from build123d import *

# Parameters (mm, degrees)
SKETCH_1_R          = 5
EXTRUDE_1_DEPTH     = 8.7
SKETCH_2_R          = 7
EXTRUDE_2_DEPTH     = 1.5
EXTRUDE_START       = -1.5
SKETCH_3_R          = 7
EXTRUDE_3_DEPTH     = 1.5
SKETCH_4_R          = 3
CUT_EXTRUDE_1_DEPTH = 10


with BuildPart() as part:
    # 草图1 → 凸台-拉伸1 (new body)
    with BuildSketch(Plane(origin=(0, 0, 0), x_dir=(0, 0, -1), z_dir=(1, 0, 0))):
        Circle(SKETCH_1_R)
    extrude(amount=EXTRUDE_1_DEPTH)

    # 草图2 → 凸台-拉伸2 (add)
    with BuildSketch(Plane(origin=(8.7, 0, 0), x_dir=(0, 0, -1), z_dir=(1, 0, 0))):
        Circle(SKETCH_2_R)
    extrude(amount=-EXTRUDE_2_DEPTH)

    # 草图3 → 凸台-拉伸3 (add)
    with BuildSketch(Plane.ZY.offset(EXTRUDE_START)):
        with Locations(Location((0, 0, 0), (0, 0, 180))):
            Circle(SKETCH_3_R)
    extrude(amount=EXTRUDE_3_DEPTH)

    # 草图4 → 切除-拉伸1 (cut)
    with BuildSketch(Plane(origin=(8.7, 0, 0), x_dir=(0, 0, -1), z_dir=(1, 0, 0))):
        Circle(SKETCH_4_R)
    extrude(amount=-CUT_EXTRUDE_1_DEPTH, mode=Mode.SUBTRACT)


solid = part.part
The listing builds one solid part. Answer for the finished solid, in the listing's coordinates (mm). A direction names the side the tool comes from. Give positions to 0.01 mm unless a question says otherwise; leave off trailing zeros. Write each loop counter-clockwise with the first axis right and the second up, starting at its lowest first coordinate (ties: lowest second). Pieces come first, ordered by that corner, then holes.
1) Section D-D (z = 3.75) is taken. Write down the section's boundary in (x, y).
2) Given P1, Ø5, axis at x = 6.5, z = 5, coming from the +Y side; P2, Ø3, axis at x = 6, y = 1.5, coming from the +Z side; P3, Ø1.5, axis at x = 2, z = 5.5, coming from the +Y side, each flat-ended and moving along its own axis, determine where each tip first touches the part or whether it passes through.
3) A tool of negligible diameter and unlimited length cuts with its end or side. For faces 4 (the face through (7.2, 5, 2)), 5 (the face through (0.76, 2.681, -6.466)), from which of +Z, -Z, +X, -X, +Y, -Y can it reach the whole face along a straight path? Write none if from no direction.
4) Section A-A (z = 0) is taken. Write down the section's boundary in (x, y), and give its area (3 significant figures).
5) Section C-C (x = 0.75) is taken. Write down the section's boundary in (y, z), and give its area (3 significant figures).
6) For a pull along Z with two mould halves and no side action, classify faces 1 (the face through (4.31, -4.88, 1.08)), 2 (the face through (4, 0, 3)), 3 (the face through (0, 3, -1)) as pulls with the +Z half, pulls with the -Z half, needs draft (parallel to the pull), parting line crosses it, or undercut.
7) Find the intervals of material crossed by L1, parallel to Y at x = 2, z = 0; L2, parallel to X at y = 5.5, z = -4; L3, parallel to Z at x = 2.75, y = 1.25, in increasing order.
Response:
1. outline: (0, -5.91) - (1.5, -5.91) - (1.5, -3.31) - (7.2, -3.31) - (7.2, -5.91) - (8.7, -5.91) - (8.7, 5.91) - (7.2, 5.91) - (7.2, 3.31) - (1.5, 3.31) - (1.5, 5.91) - (0, 5.91) - close
2. P1: stops at y = 6.5
2. P2: stops at z = 6.97
2. P3: stops at y = 4.96
3. face 4: none
3. face 5: +X, -X
4. outline: (0, -7) - (1.5, -7) - (1.5, -5) - (7.2, -5) - (7.2, -7) - (8.7, -7) - (8.7, -3) - (0, -3) - close; (0, 3) - (8.7, 3) - (8.7, 7) - (7.2, 7) - (7.2, 5) - (1.5, 5) - (1.5, 7) - (0, 7) - close
4. area: 46.8 mm2
5. outline: circle Ø14 at (0, 0); hole circle Ø6 at (0, 0)
5. area: 126 mm2
6. face 1: parting line crosses it
6. face 2: undercut
6. face 3: needs draft
7. L1: y = -5 to -3, 3 to 5
7. L2: x = 0 to 1.5, 7.2 to 8.7
7. L3: z = -4.84 to -2.73, 2.73 to 4.84
